```python
from build123d import *

# Parameters (mm, degrees)
PAD_DEPTH    = 1
PAD004_DEPTH = 20
FILLET_R     = 10
FILLET001_R  = 2


with BuildPart() as part:
    # Sketch → Pad (new body)
    with BuildSketch(Plane.XY):
        with BuildLine():
            ThreePointArc((0, 65), (-39.250322, 51.811314), (-62.572638, 17.5973))
            ThreePointArc((-62.572638, 17.5973), (-62.281657, 16.256919), (-61.1956, 15.4192))
            Line((-61.1956, 15.4192), (-48.0942, 15.4192))
            ThreePointArc((-48.0942, 15.4192), (-46.017568, 16.268418), (-44.521334, 17.9402))
            ThreePointArc((44.629065, 17.6705), (0.14521, 47.99978), (-44.521334, 17.9402))
            ThreePointArc((44.629065, 17.6705), (45.695788, 16.297968), (47.167959, 15.3736))
            Line((47.167959, 15.3736), (54.923211, 15.384158))
            ThreePointArc((54.923211, 15.384158), (76.110008, 24.185371), (84.88237, 45.38413))
            Line((84.88237, 59.61183), (84.88237, 45.38413))
            ThreePointArc((84.88237, 59.61183), (83.304212, 63.421842), (79.4942, 65))
            Line((0, 65), (79.4942, 65))
        make_face()
    extrude(amount=PAD_DEPTH)

    # Sketch001 → Pad004 (new body)
    with BuildSketch(Plane.XY.offset(1)):
        with BuildLine():
            ThreePointArc((6e-05, 65), (-39.693641, 51.472467), (-62.865542, 16.5204))
            Line((-62.865542, 16.5204), (-59.765542, 16.5204))
            ThreePointArc((6e-05, 63), (-37.80132, 49.942273), (-59.765542, 16.5204))
            Line((80.00006, 63), (6e-05, 63))
            Line((80.00006, 65), (80.00006, 63))
            Line((6e-05, 65), (80.00006, 65))
        make_face()
    extrude(amount=PAD004_DEPTH)

    # Fillet
    fillet_edges = [part.edges().sort_by_distance(p)[0] for p in [
        (80.00006, 64, 21),
    ]]
    fillet(fillet_edges, radius=FILLET_R)

    # Fillet001
    fillet001_edges = [part.edges().sort_by_distance(p)[0] for p in [
        (-61.315542, 16.5204, 21),
    ]]
    fillet(fillet001_edges, radius=FILLET001_R)


solid = part.part
```
Verification items for the finished model (mm, model axes). A direction names the side the tool comes from. Give positions to 0.01 mm unless a question says otherwise; leave off trailing zeros. Order: outer loops, then holes, each group sorted by start corner. A loop starts at its lowest first (then second) coordinate and runs counter-clockwise, first axis right, second up. Notation, with made-up numbers: M -4,49.25 L 3,49.25 A15 cw 3,70.25 Z; hole C -2,89.25 d5. An arc over 180 degrees is marked long. Answer in a Markdown table with one row per item. Add a question column.
Item 1: Scan lines: probe 1 along Y at (x, z) = (79, 2); probe 2 along Z at (x, y) = (65, 47); probe 3 along X at (y, z) = (18.5, 9). Record each from-to range of solid material in increasing order. Write a range as from..to.
Item 2: Section check B-B, the plane x = -30. Enter the section's corners in (y, z), and give its area (3 significant figures).
Item 3: Section check C-C, the plane z = 16.5. Enter the section's corners in (x, y), and give its area (3 significant figures).
Item 4: Section check D-D, the plane y = 57. Enter the section's corners in (x, z).
Item 5: Tool access check on faces 1 (the flat face through (-61, 16.52, 10)), 2 (the cylindrical face through (-37.35, 50.29, 10.86)), 3 (the cylindrical face through (76.99, 63.99, 18.15)). Record the directions out of +Z, -Z, +X, -X, +Y, -Y that give a thin tool (end or side, any length) a straight path to the whole face; none if there is none.
Item 6: Mould release check, pull along X, two halves, no side actions. Record for faces 4 (the cylindrical face through (-46.044, 16.25, 0.493)), 5 (the flat face through (41, 63, 11)), 6 (the cylindrical face through (83.346, 63.38, 0.493)): released by +X, released by -X, zero draft, split by the parting line, or undercut.
Item 7: Gauge pin test, flat ends, axial feed: pin 1 (1 mm diameter, centred on y = 64.5, z = 7.5, fed in from +X); pin 2 (0.5 mm diameter, centred on x = -51.5, z = 0.5, fed in from -Y); pin 3 (1.5 mm diameter, centred on x = 50.5, z = 3, fed in from -Y). Record the tip position at first contact, or that the pin passes through.
Item 8: Section check A-A, the plane y = 26.5. Enter the section's corners in (x, z).
Filled sheet:
| question | item | result |
|---|---|---|
| 1 | probe 1 | y = 63..65 |
| 1 | probe 2 | z = 0..1 |
| 1 | probe 3 | x = -62.31..-59.22 |
| 2 | outline | M 37.47,0 L 57.66,0 L 57.66,21 L 55.11,21 L 55.11,1 L 37.47,1 Z |
| 2 | area | 71.2 mm^2 |
| 3 | outline | M -62.87,16.52 L -59.77,16.52 A62 cw 0,63 L 78.35,63 L 78.35,65 L 0,65 A65 ccw Z |
| 3 | area | 358 mm^2 |
| 4 | outline | M -31.24,0 L 84.88,0 L 84.88,1 L -26.35,1 L -26.35,21 L -31.24,21 Z |
| 5 | face 1 | +Z, +X, -X, -Y |
| 5 | face 2 | +Z, +X, -Y |
| 5 | face 3 | +Z, +X, +Y, -Y |
| 6 | face 4 | undercut |
| 6 | face 5 | zero draft |
| 6 | face 6 | released by +X |
| 7 | pin 1 | stops at x = 80 |
| 7 | pin 2 | stops at y = 15.42 |
| 7 | pin 3 | stops at y = 63 |
| 8 | outline | M -59.35,0 L -40.02,0 L -40.02,1 L -56.25,1 L -56.25,21 L -59.35,21 Z; M 40.02,0 L 78.19,0 L 78.19,1 L 40.02,1 Z |
